```python
from build123d import *

# Parameters (mm, degrees)
SKETCH_W               = 100
SKETCH_H               = 110
PAD_DEPTH              = 10
SKETCH001_R            = 2.5
HOLE_DEPTH             = 10.001
LINEARPATTERN_COUNT    = 2
LINEARPATTERN_PITCH    = 55
HOLE001_D              = 8.8
HOLE001_CSINK_D        = 16
HOLE001_CSINK_ANGLE    = 90
LINEARPATTERN001_COUNT = 2
LINEARPATTERN001_PITCH = 40
HOLE002_D              = 8.8
HOLE002_CSINK_D        = 16
HOLE002_CSINK_ANGLE    = 90
LINEARPATTERN002_COUNT = 2
LINEARPATTERN002_PITCH = 40


with BuildPart() as part:
    # Sketch → Pad (new body)
    with BuildSketch(Plane.XY):
        with Locations((50, 55)):
            Rectangle(SKETCH_W, SKETCH_H)
    extrude(amount=PAD_DEPTH)

    # Sketch001 (on Face6 of Pad) → Hole (cut, through all)
    with BuildSketch(Plane.XY.offset(10)):
        with Locations((9, 8)):
            Circle(SKETCH001_R)
    hole = extrude(amount=-HOLE_DEPTH, mode=Mode.SUBTRACT)

    # LinearPattern: Hole ×2
    with Locations(*[(0, i * LINEARPATTERN_PITCH, 0) for i in range(1, LINEARPATTERN_COUNT)]):
        add(hole, mode=Mode.SUBTRACT)

    # Hole001 (through all)
    with Locations(Plane.XY.offset(10)):
        with Locations((80, 20)):
            hole001 = CounterSinkHole(HOLE001_D / 2, HOLE001_CSINK_D / 2, counter_sink_angle=HOLE001_CSINK_ANGLE)

    # LinearPattern001: Hole001 ×2
    with Locations(*[(0, i * LINEARPATTERN001_PITCH, 0) for i in range(1, LINEARPATTERN001_COUNT)]):
        add(hole001, mode=Mode.SUBTRACT)

    # Hole002 (through all)
    with Locations(Plane.XY.offset(10)):
        with Locations((30, 90)):
            hole002 = CounterSinkHole(HOLE002_D / 2, HOLE002_CSINK_D / 2, counter_sink_angle=HOLE002_CSINK_ANGLE)

    # LinearPattern002: Hole002 ×2
    with Locations(*[(i * LINEARPATTERN002_PITCH, 0, 0) for i in range(1, LINEARPATTERN002_COUNT)]):
        add(hole002, mode=Mode.SUBTRACT)


solid = part.part
```
Here's how the part is built. I have some questions about the finished solid (model axes, mm). Round coordinates to 2 decimals unless told otherwise and drop trailing zeros. Loops run counter-clockwise (first coordinate to the right, second up) from the corner with the lowest first, then second, coordinate; pieces in that order, holes last.
1. Suppose I cut it at D-D, the plane x = 80. Please give me the cut outline in (y, z), and give its area (3 significant figures).
Answers:
outline: (0, 0) - (15.6, 0) - (15.6, 6.4) - (12, 10) - (0, 10) - close; (24.4, 0) - (55.6, 0) - (55.6, 6.4) - (52, 10) - (28, 10) - (24.4, 6.4) - close; (64.4, 0) - (110, 0) - (110, 10) - (68, 10) - (64.4, 6.4) - close
area: 898 mm2
2. Will these pins go through, and if not, where does the flat tip stop? pin 1 (5.5 mm diameter, centred on x = 70, y = 90, fed in from +Z); pin 2 (11.5 mm diameter, centred on x = 30, y = 90, fed in from +Z).
Answers:
pin 1: passes through
pin 2: stops at z = 7.75
3. Suppose I cut it at B-B, the plane y = 8. Please give me the cut outline in (x, z).
Answers:
outline: (0, 0) - (6.5, 0) - (6.5, 10) - (0, 10) - close; (11.5, 0) - (100, 0) - (100, 10) - (11.5, 10) - close
4. If I drill on probe 1 along Y at (x, z) = (9, 5.5); probe 2 along X at (y, z) = (90, 2); probe 3 along Y at (x, z) = (80, 2.5), over which ranges is the centre line in solid material (lowest first)?
Answers:
probe 1: y = 0 to 5.5, 10.5 to 60.5, 65.5 to 110
probe 2: x = 0 to 25.6, 34.4 to 65.6, 74.4 to 100
probe 3: y = 0 to 15.6, 24.4 to 55.6, 64.4 to 110
5. Suppose I cut it at C-C, the plane z = 8. Please give me the cut outline in (x, y).
Answers:
outline: (0, 0) - (100, 0) - (100, 110) - (0, 110) - close; hole circle Ø5 at (9, 8); hole circle Ø5 at (9, 63); hole circle Ø12 at (30, 90); hole circle Ø12 at (70, 90); hole circle Ø12 at (80, 20); hole circle Ø12 at (80, 60)
6. Thinking about a two-plate mould opening in X: for faces 1 (the face through (8.67, 65.48, 5.07)), 2 (the face through (49, 56, 10)), 3 (the face through (0, 54, 5)), 4 (the face through (100, 54, 5)), which applies, released by +X, released by -X, zero draft, split by the parting line, or undercut?
Answers:
face 1: undercut
face 2: zero draft
face 3: released by -X
face 4: released by +X
7. Suppose I cut it at A-A, the plane x = 70. Please give me the cut outline in (y, z).
Answers:
outline: (0, 0) - (85.6, 0) - (85.6, 6.4) - (82, 10) - (0, 10) - close; (94.4, 0) - (110, 0) - (110, 10) - (98, 10) - (94.4, 6.4) - close
